Study the drawing (mm; zero at the part's minimum x, y, z) and answer. A direction names the side the tool comes from. Coordinates: 2 decimals unless noted, no trailing zeros. Order: outer loops, then holes, each group sorted by start corner. A loop starts at its lowest first (then second) coordinate and runs counter-clockwise, first axis right, second up. Notation, with made-up numbers: (-6.75, -0.75) -> (10.25, -0.75) arc R15 ccw to (10.25, 25.25) -> close; hole circle Ø11 at (16, -27.5). An arc over 180 degrees is marked (long way). Answer in a Markdown table with one row per item. Add a question column.
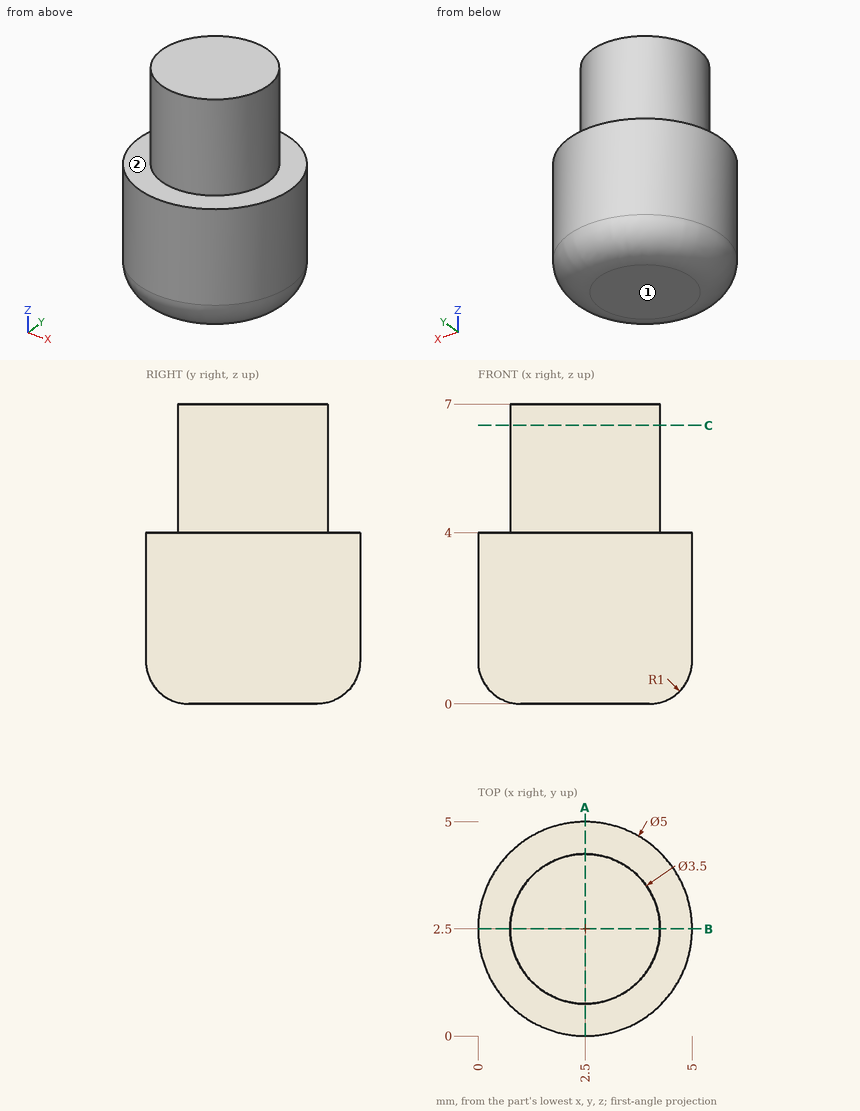
Q1. For the marked faces 1 and 2, determine the directions among +Z, -Z, +X, -X, +Y, -Y from which every point of the face is accessible in a straight line to the end or side of a thin tool.
Q2. Given pin 1 (1.5 mm diameter, centred on y = 3.5, z = 1.5, fed in from +X); pin 2 (3 mm diameter, centred on x = 3, y = 0.5, fed in from +Z); pin 3 (1.5 mm diameter, centred on y = 0.5, z = 2.5, fed in from +X), each flat-ended and moving along its own axis, determine where each tip first touches the part or whether it passes through.
Q3. Straight lines are drawn through the part: line 1 (Z direction, x = 2, y = 4.45); line 2 (X direction, y = 3.7, z = 1.25); line 3 (X direction, y = 3.1, z = 5.75). For each, find the intervals that lie inside material, in ascending order.
Q4. A cutting plane is placed at C-C (z = 6.5). Determine the outline of the cut face in (x, y), then the cut area to 3 significant figures.
Q5. A cutting plane is placed at A-A (x = 2.5). Determine the outline of the cut face in (y, z).
Returned:
| question | item | result |
|---|---|---|
| 1 | face 1 | -Z, +X, -X, +Y, -Y |
| 1 | face 2 | +Z |
| 2 | pin 1 | stops at x = 4.99 |
| 2 | pin 2 | stops at z = 7 |
| 2 | pin 3 | stops at x = 4.67 |
| 3 | line 1 | z = 0.14 to 4 |
| 3 | line 2 | x = 0.31 to 4.69 |
| 3 | line 3 | x = 0.86 to 4.14 |
| 4 | outline | circle Ø3.5 at (2.5, 2.5) |
| 4 | area | 9.62 mm² |
| 5 | outline | (0, 1) arc R1 ccw to (1, 0) -> (4, 0) arc R1 ccw to (5, 1) -> (5, 4) -> (4.25, 4) -> (4.25, 7) -> (0.75, 7) -> (0.75, 4) -> (0, 4) -> close |
